Verification items for the finished model (mm, model axes). A direction names the side the tool comes from. Coordinates: 2 decimals unless noted, no trailing zeros. Order: outer loops, then holes, each group sorted by start corner. A loop starts at its lowest first (then second) coordinate and runs counter-clockwise, first axis right, second up. Notation, with made-up numbers: M 52.25,53 L 67.25,53 A17 cw 67.25,86 Z; hole C 22,70.25 d3. An arc over 180 degrees is marked long. Return JSON: item names as keys, results as strings. Group by question number.
1. Section check A-A, the plane x = 0. Record the cut outline in (y, z) (3 decimals).
2. Section check B-B, the plane z = 0. Record the cut outline in (x, y) (3 decimals), plus the area to 3 significant figures.
3. Mould release check, pull along Z, two halves, no side actions. Record for faces 4 (the cylindrical face through (7.62, 23.31, 3.16)), 5 (the cylindrical face through (2.58, 24.08, -4.05)), 6 (the flat face through (1, 22.3, -6)): +Z half, -Z half, draft (parallel to the pull), parting line (faces both ways), or undercut.
4. Gauge pin test, flat ends, axial feed: pin 1 (4 mm diameter, centred on x = -4.5, y = 33.5, fed in from +Z); pin 2 (1.5 mm diameter, centred on y = 11.5, z = 2, fed in from -X); pin 3 (2 mm diameter, centred on y = 24.5, z = 4.5, fed in from +X). Record the tip position at first contact, or that the pin passes through.
5. Set-up check for faces 1 (the flat face through (-1, 37.3, 5)), 2 (the cylindrical face through (-0.75, 15.5, -5.7)), 3 (the flat face through (-1, 24.3, -6)): record each of +Z, -Z, +X, -X, +Y, -Y from which the full face is reachable in a straight line by a thin tool's end or side.
6. Material ranges on line 1 along Z through (x, y) = (0, 31); line 2 along Y through (x, z) = (-3.5, 6), recorded low to high.
7. Section check C-C, the plane y = 21.5. Record the cut outline in (x, z).
```python
from build123d import *


with BuildPart() as part:
    # Sketch1 → 5.63 mm bottom to pen tip (revolve)
    with BuildSketch(Plane.XY):
        Polygon((0, 0), (2.375, 0), (3.2, 5.5), (3.2, 6.5), (4.75, 6.5), (5.75, 8.5), (5.75, 22.3), (7, 22.3), (8.25, 22.55), (8.25, 24.05), (7, 24.3), (5.75, 24.3), (5.75, 37.3), (0, 37.3), align=None)
    revolve(axis=Axis((0, -143.950460456, 0), (0, 1, 0)))

    # Sketch2 → Cut-Revolve1 (revolve, cut)
    with BuildSketch(Plane.XY):
        Polygon((0, -5.63), (0.39, -5.63), (0.39, -2.03), (1.1, -2.03), (1.65, 0.35), (2.4, 0.35), (4.185, 10.48), (4.8, 10.48), (4.8, 42.48), (5.967443991, 42.48), (5.967443991, 45.051498483), (0, 45.051498483), align=None)
    revolve(axis=Axis((0, -1000, 0), (0, 1, 0)), mode=Mode.SUBTRACT)


with BuildPart() as body_2:
    # of the pieces the cut leaves, the one that is kept (cut_revolve1_keep)
    add(part.part.solids().sort_by_distance((4.75, 6.5, 0))[0])


solid = body_2.part
```
Answers follow:
{
 "1": {"outline": "M 6.5,-4.75 L 8.5,-5.75 L 22.3,-5.75 L 22.3,-7 L 22.55,-8.25 L 24.05,-8.25 L 24.3,-7 L 24.3,-5.75 L 37.3,-5.75 L 37.3,-4.8 L 10.48,-4.8 L 10.48,-4.185 L 6.5,-3.484 Z; M 6.5,3.484 L 10.48,4.185 L 10.48,4.8 L 37.3,4.8 L 37.3,5.75 L 24.3,5.75 L 24.3,7 L 24.05,8.25 L 22.55,8.25 L 22.3,7 L 22.3,5.75 L 8.5,5.75 L 6.5,4.75 Z"},
 "2": {"outline": "M -8.25,22.55 L -7,22.3 L -5.75,22.3 L -5.75,8.5 L -4.75,6.5 L -3.484,6.5 L -4.185,10.48 L -4.8,10.48 L -4.8,37.3 L -5.75,37.3 L -5.75,24.3 L -7,24.3 L -8.25,24.05 Z; M 3.484,6.5 L 4.75,6.5 L 5.75,8.5 L 5.75,22.3 L 7,22.3 L 8.25,22.55 L 8.25,24.05 L 7,24.3 L 5.75,24.3 L 5.75,37.3 L 4.8,37.3 L 4.8,10.48 L 4.185,10.48 Z", "area": "73.6 mm^2"},
 "3": {"face 4": "parting line", "face 5": "undercut", "face 6": "draft"},
 "4": {"pin 1": "z = 5.18", "pin 2": "x = -5.61", "pin 3": "x = 7.42"},
 "5": {"face 1": "+Z, -Z, +X, -X, +Y", "face 2": "-Y", "face 3": "+Y"},
 "6": {"line 1": "-5.75 to -4.8, 4.8 to 5.75", "line 2": "22.3 to 24.3"},
 "7": {"outline": "C 0,0 d11.5; hole C 0,0 d9.6"}
}
